Verification items for the finished model (mm, model axes). A direction names the side the tool comes from. Round coordinates to 2 decimals unless told otherwise and drop trailing zeros. Order: outer loops, then holes, each group sorted by start corner. A loop starts at its lowest first (then second) coordinate and runs counter-clockwise, first axis right, second up. Notation, with made-up numbers: (88.5, 63) -> (100.5, 63) arc R16 cw to (100.5, 80) -> close; hole circle Ø5 at (1, 82.25). An arc over 180 degrees is marked (long way). Put each result on its own line as item: value.
from build123d import *

# Parameters (mm, degrees)
SKETCH1_W           = 16.3
SKETCH1_H           = 16.3
SKETCH1_W_2         = 11
SKETCH1_H_2         = 11
SKETCH1_R           = 2.6
BOSS_EXTRUDE1_DEPTH = 200
CUT_EXTRUDE2_DEPTH  = 201.499376558
FILLET1_R           = 2.5
FILLET2_R           = 2.5
SKETCH3_W           = 1
SKETCH3_H           = 7.25
SKETCH3_W_2         = 7.25
SKETCH3_H_2         = 1
CUT_EXTRUDE3_DEPTH  = 201.499376558


with BuildPart() as part:
    # Sketch1 → Boss-Extrude1 (new body)
    # profile 1 of 6: a face of its own
    with BuildSketch(Plane.XY):
        Polygon((-3.1, 8.15), (-3.1, 10), (-10, 10), (-10, 3.1), (-8.15, 3.1), (-8.15, 8.15), align=None)
    # profile 2 of 6: a face of its own
    with BuildSketch(Plane.XY):
        Polygon((10, 10), (3.1, 10), (3.1, 8.15), (8.15, 8.15), (8.15, 3.1), (10, 3.1), align=None)
    # profile 3 of 6: a face of its own
    with BuildSketch(Plane.XY):
        Rectangle(SKETCH1_W, SKETCH1_H)
        Rectangle(SKETCH1_W_2, SKETCH1_H_2, mode=Mode.SUBTRACT)
    # profile 4 of 6: a face of its own
    with BuildSketch(Plane.XY):
        Polygon((10, -10), (10, -3.1), (8.15, -3.1), (8.15, -8.15), (3.1, -8.15), (3.1, -10), align=None)
    # profile 5 of 6: a face of its own
    with BuildSketch(Plane.XY):
        Polygon((-8.15, -3.1), (-10, -3.1), (-10, -10), (-3.1, -10), (-3.1, -8.15), (-8.15, -8.15), align=None)
    # profile 6 of 6: a face of its own
    with BuildSketch(Plane.XY):
        Rectangle(SKETCH1_W_2, SKETCH1_H_2)
        Circle(SKETCH1_R, mode=Mode.SUBTRACT)
    extrude(amount=BOSS_EXTRUDE1_DEPTH)

    # Sketch2 → Cut-Extrude2 (cut, through all)
    with BuildSketch(Plane.XY.offset(200)):
        Polygon((-5.5, -4.580761184), (-5.5, 4.580761184), (-6.419238816, 5.5), (-7.6, 5.5), (-8.15, 4.95), (-8.15, 3.1), (-8.15, -3.1), (-8.15, -4.95), (-7.6, -5.5), (-6.419238816, -5.5), align=None)
        Polygon((-3.9, -2.980761184), (-3.9, 2.980761184), (-5.5, 4.580761184), (-5.5, -4.580761184), align=None)
        Polygon((-5.5, 6.419238816), (-4.580761184, 5.5), (4.580761184, 5.5), (5.5, 6.419238816), (5.5, 7.6), (4.95, 8.15), (3.1, 8.15), (-3.1, 8.15), (-4.95, 8.15), (-5.5, 7.6), align=None)
        Polygon((-4.580761184, 5.5), (-2.980761184, 3.9), (2.980761184, 3.9), (4.580761184, 5.5), align=None)
        Polygon((6.419238816, 5.5), (5.5, 4.580761184), (5.5, -4.580761184), (6.419238816, -5.5), (7.6, -5.5), (8.15, -4.95), (8.15, -3.1), (8.15, 3.1), (8.15, 4.95), (7.6, 5.5), align=None)
        Polygon((5.5, 4.580761184), (3.9, 2.980761184), (3.9, -2.980761184), (5.5, -4.580761184), align=None)
        Polygon((4.580761184, -5.5), (-4.580761184, -5.5), (-5.5, -6.419238816), (-5.5, -7.6), (-4.95, -8.15), (-3.1, -8.15), (3.1, -8.15), (4.95, -8.15), (5.5, -7.6), (5.5, -6.419238816), align=None)
        Polygon((2.980761184, -3.9), (-2.980761184, -3.9), (-4.580761184, -5.5), (4.580761184, -5.5), align=None)
    extrude(amount=-CUT_EXTRUDE2_DEPTH, mode=Mode.SUBTRACT)

    # Fillet1
    fillet1_edges = [part.edges().sort_by_distance(p)[0] for p in [
        (-10, -10, 100),
        (-10, 10, 100),
        (10, 10, 100),
        (10, -10, 100),
    ]]
    fillet(fillet1_edges, radius=FILLET1_R)

    # Fillet2
    fillet2_edges = [part.edges().sort_by_distance(p)[0] for p in [
        (2.980761184, 3.9, 100),
        (3.9, -2.980761184, 100),
        (-2.980761184, -3.9, 100),
        (2.980761184, -3.9, 100),
        (-3.9, 2.980761184, 100),
        (-3.9, -2.980761184, 100),
    ]]
    fillet(fillet2_edges, radius=FILLET2_R)

    # Sketch3 → Cut-Extrude3 (cut, through all)
    with BuildSketch(Plane.XY.offset(200)):
        with Locations((10, 0)):
            Rectangle(SKETCH3_W, SKETCH3_H)
        with Locations((0, 10)):
            Rectangle(SKETCH3_W_2, SKETCH3_H_2)
        with Locations((0, -10)):
            Rectangle(SKETCH3_W_2, SKETCH3_H_2)
        with Locations((-10, 0)):
            Rectangle(SKETCH3_W, SKETCH3_H)
    extrude(amount=-CUT_EXTRUDE3_DEPTH, mode=Mode.SUBTRACT)


solid = part.part
Item 1: Section check A-A on x = 0. Record the boundary of the cut face in (y, z).
Check sheet entries:
outline: (-3.9, 0) -> (-2.6, 0) -> (-2.6, 200) -> (-3.9, 200) -> close; (2.6, 0) -> (3.9, 0) -> (3.9, 200) -> (2.6, 200) -> close
Item 2: Release check for a two-part mould opening along X. For faces 1 (the flat face through (-1, 3.9, 101)), 2 (the flat face through (-6, -10, 99)), 3 (the flat face through (-10, 6, 99)) record: +X half, -X half, draft (parallel to the pull), parting line (faces both ways), or undercut.
Check sheet entries:
face 1: undercut
face 2: draft
face 3: -X half
Item 3: Gauge pin test, flat ends, axial feed: pin 1 Ø1.5 at (y, z) = (1.5, 103) entering from +X; pin 2 Ø0.7 at (x, z) = (-9, 143) entering from -Y; pin 3 Ø5.5 at (x, z) = (0, 132) entering from +Y. Record the tip position at first contact, or that the pin passes through.
Check sheet entries:
pin 1: stops at x = 3.9
pin 2: stops at y = -9.72
pin 3: stops at y = 4.03
Item 4: Material ranges on L1, parallel to Y at x = 0, z = 88; L2, parallel to X at y = -1.75, z = 174.5; L3, parallel to X at y = -7.5, z = 112.5, recorded low to high. Write a range as [from, to].
Check sheet entries:
L1: y = [-3.9, -2.6], [2.6, 3.9]
L2: x = [-3.9, -1.92], [1.92, 3.9]
L3: x = [-10, -5.5], [5.5, 10]
Item 5: Tool access check on faces 4 (the flat face through (-3.9, 0, 101)), 5 (the flat face through (3.9, 1, 101)), 6 (the flat face through (0, -3.9, 101)), 7 (the flat face through (10, -6, 99)). Record the directions out of +Z, -Z, +X, -X, +Y, -Y that give a thin tool (end or side, any length) a straight path to the whole face; none if there is none.
Check sheet entries:
face 4: +Z, -Z, -X
face 5: +Z, -Z, +X
face 6: +Z, -Z, -Y
face 7: +Z, -Z, +X, +Y, -Y
